Can you work these out from the drawing? Everything is in mm from the part's minimum corner. Give positions to 0.01 mm unless a question says otherwise; leave off trailing zeros. Write each loop counter-clockwise with the first axis right and the second up, starting at its lowest first coordinate (ties: lowest second). Pieces come first, ordered by that corner, then holes. Notation, with made-up numbers: (36, 45) - (52, 45) arc R28 cw to (52, 67) - close; hole circle Ø6 at (8.5, 4). An arc over 180 degrees is marked (long way). Answer in a Markdown table with one row per item.
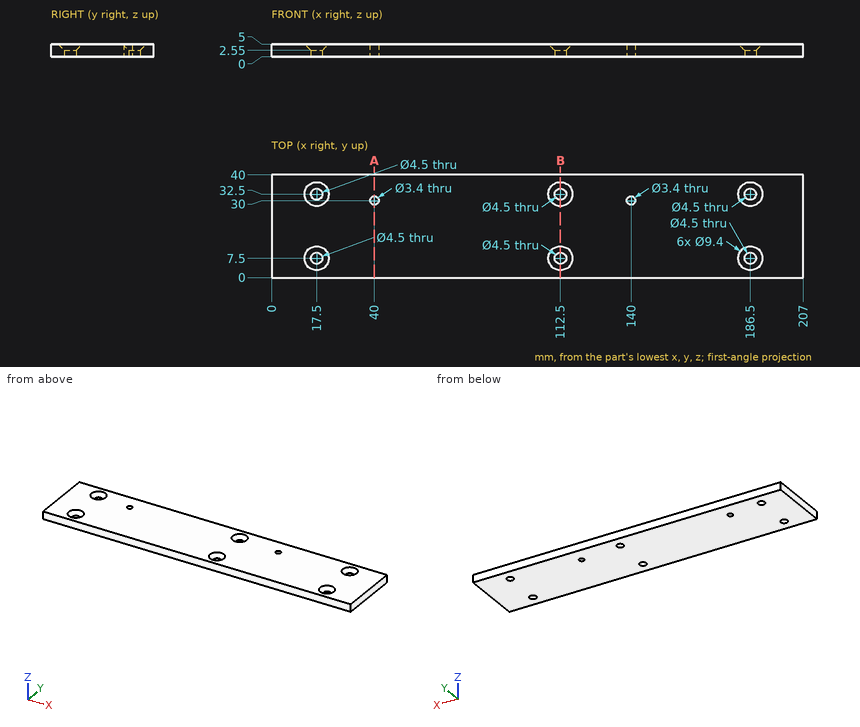
1) If I drill on line 1 (Y direction, x = 112.5, z = 1.35); line 2 (X direction, y = 7.5, z = 1.15); line 3 (X direction, y = 6, z = 0.3), over which ranges is the centre line in solid material (lowest first)?
Check values:
| item | result |
|---|---|
| line 1 | y = 0 to 5.25, 9.75 to 30.25, 34.75 to 40 |
| line 2 | x = 0 to 15.25, 19.75 to 110.25, 114.75 to 184.25, 188.75 to 207 |
| line 3 | x = 0 to 15.82, 19.18 to 110.82, 114.18 to 184.82, 188.18 to 207 |
2) Imagine slicing it at A-A (x = 40). List the corners of the cut face in (y, z) for me, then the cut area to 3 significant figures.
Check values:
| item | result |
|---|---|
| outline | (0, 0) - (28.3, 0) - (28.3, 5) - (0, 5) - close; (31.7, 0) - (40, 0) - (40, 5) - (31.7, 5) - close |
| area | 183 mm2 |
3) Imagine slicing it at B-B (x = 112.5). List the corners of the cut face in (y, z) for me.
Check values:
| item | result |
|---|---|
| outline | (0, 0) - (5.25, 0) - (5.25, 2.55) - (2.8, 5) - (0, 5) - close; (9.75, 0) - (30.25, 0) - (30.25, 2.55) - (27.8, 5) - (12.2, 5) - (9.75, 2.55) - close; (34.75, 0) - (40, 0) - (40, 5) - (37.2, 5) - (34.75, 2.55) - close |
4) Will these pins go through, and if not, where does the flat tip stop? P1, Ø5, axis at x = 17.5, y = 7.5, coming from the +Z side; P2, Ø7, axis at x = 112.5, y = 7.5, coming from the +Z side.
Check values:
| item | result |
|---|---|
| P1 | stops at z = 2.8 |
| P2 | stops at z = 3.8 |
